Check sheet for the modelled part. Datum: model origin and axes. Units: mm. Face numbers are marked on the shaded views. A direction names the side the tool comes from. Round coordinates to 2 decimals unless told otherwise and drop trailing zeros. Order: outer loops, then holes, each group sorted by start corner. A loop starts at its lowest first (then second) coordinate and runs counter-clockwise, first axis right, second up.
(1) Sectioned sample at B-B, the plane x = 0. Enter the section's corners in (y, z), and give its area (3 significant figures).
(2) Thickness scan on probe 1 along Z at (x, y) = (35, 4.1); probe 2 along X at (y, z) = (4, 12.75); probe 3 along Z at (x, y) = (0, -5.2). Record the ranges inside material, lowest first.
(3) Depth check by flat-ended pin: pin 1 (2 mm diameter, centred on y = -3, z = 2.5, fed in from +X); pin 2 (4 mm diameter, centred on x = 32.5, z = 13, fed in from -Y); pin 3 (1 mm diameter, centred on x = 23.5, y = 0.5, fed in from -Z); pin 4 (1.5 mm diameter, centred on y = -3, z = 4.5, fed in from -X). Enter the tip coordinate at first touch or a pass-through.
(4) Sectioned sample at D-D, the plane z = 2.25. Enter the section's corners in (x, y), and give its area (3 significant figures).
(5) Mould release check, pull along Z, two halves, no side actions. Record for the marked faces 4, 5 and 6: released by +Z, released by -Z, zero draft, split by the parting line, or undercut.
(6) Sectioned sample at A-A, the plane z = 10. Count the separate pieces of the cut face and the enclosed holes in it, and give its area (3 significant figures).
(7) Tool access check on the marked faces 1, 2 and 3. Record the directions out of +Z, -Z, +X, -X, +Y, -Y that give a thin tool (end or side, any length) a straight path to the whole face; none if there is none.
(8) Sectioned sample at C-C, the plane y = -5. Enter the section's corners in (x, z), and give its area (3 significant figures).
```python
from build123d import *

# Parameters (mm, degrees)
F0_W     = 10
F0_H     = 5
F1_DEPTH = 20
F2_R     = 3.15
F3_DEPTH = 25
F4_R     = 2.65
F5_DEPTH = 25
F6_R     = 1.5


with BuildPart() as f1:
    # F0 (on Top) → F1 (new body)
    with BuildSketch(Plane.XY):
        with Locations((-35, 5)):
            Rectangle(F0_W, F0_H)
        Polygon((30, 2.5), (30, 7.5), (25, 7.5), (25, -2.5), (-25, -2.5), (-25, 7.5), (-30, 7.5), (-30, 2.5), (-30, -7.5), (30, -7.5), align=None)
        with Locations((35, 5)):
            Rectangle(F0_W, F0_H)
    extrude(amount=F1_DEPTH)

    # F2 (on face) → F3 (cut)
    with BuildSketch(Plane.XZ.offset(7.5)):
        with Locations((0, 10)):
            Circle(F2_R)
    extrude(amount=-F3_DEPTH, mode=Mode.SUBTRACT)

    # F4 (on face) → F5 (cut)
    with BuildSketch(Plane.XZ.offset(-2.5)):
        with Locations((-35, 10)):
            Circle(F4_R)
        with Locations((35, 10)):
            Circle(F4_R)
    extrude(amount=-F5_DEPTH, mode=Mode.SUBTRACT)

    # F6
    f6_edges = [f1.edges().sort_by_distance(p)[0] for p in [
        (-25, -2.5, 10),
        (25, -2.5, 10),
        (40, 7.5, 10),
        (40, 2.5, 10),
        (30, -7.5, 10),
        (-30, -7.5, 10),
        (-40, 2.5, 10),
        (-40, 7.5, 10),
        (-25, 7.5, 10),
        (25, 7.5, 10),
    ]]
    fillet(f6_edges, radius=F6_R)


solid = f1.part
```
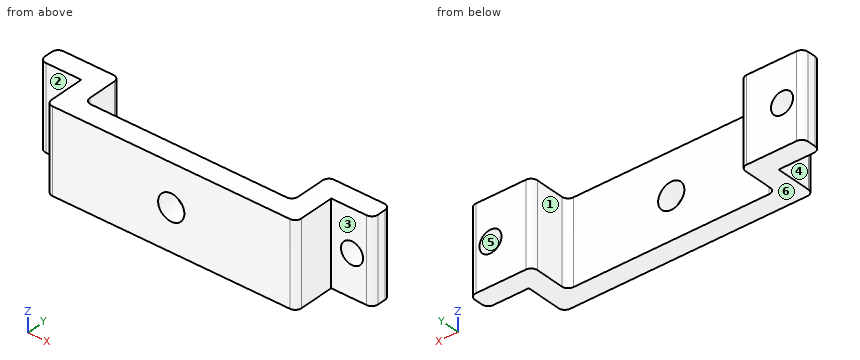
Derived:
1. outline: (-7.5, 0) - (-2.5, 0) - (-2.5, 6.85) - (-7.5, 6.85) - close; (-7.5, 13.15) - (-2.5, 13.15) - (-2.5, 20) - (-7.5, 20) - close
1. area: 68.5 mm2
2. probe 1: z = 0 to 7.35, 12.65 to 20
2. probe 2: x = -40 to -25, 25 to 40
2. probe 3: z = 0 to 6.85, 13.15 to 20
3. pin 1: stops at x = 30
3. pin 2: stops at y = 2.5
3. pin 3: passes through
3. pin 4: stops at x = -30
4. outline: (-40, 4) arc R1.5 ccw to (-38.5, 2.5) - (-30, 2.5) - (-30, -6) arc R1.5 ccw to (-28.5, -7.5) - (28.5, -7.5) arc R1.5 ccw to (30, -6) - (30, 2.5) - (38.5, 2.5) arc R1.5 ccw to (40, 4) - (40, 6) arc R1.5 ccw to (38.5, 7.5) - (26.5, 7.5) arc R1.5 ccw to (25, 6) - (25, -1) arc R1.5 cw to (23.5, -2.5) - (-23.5, -2.5) arc R1.5 cw to (-25, -1) - (-25, 6) arc R1.5 ccw to (-26.5, 7.5) - (-38.5, 7.5) arc R1.5 ccw to (-40, 6) - close
4. area: 497 mm2
5. face 4: zero draft
5. face 5: undercut
5. face 6: released by -Z
6. separate pieces: 4
6. enclosed holes: 0
6. area: 413 mm2
7. face 1: +Z, -Z, +Y
7. face 2: +Z, -Z, -X, -Y
7. face 3: +Z, -Z, +X, -Y
8. outline: (-30, 0) - (30, 0) - (30, 20) - (-30, 20) - close; hole circle Ø6.3 at (0, 10)
8. area: 1,170 mm2
